```python
from build123d import *

# Parameters (mm, degrees)
F1_DEPTH = 30
F2_R     = 4.4
F3_R     = 4.4
F4_DEPTH = 25
F5_R     = 2
F6_R     = 2


# Not quite as in the source:
# - a feature names something its author has since deleted; it is built from what else it names


with BuildPart() as f1:
    # F0 (on Front) → F1 (new body)
    with BuildSketch(Plane.XZ):
        Polygon((90, -1), (90, 1), (70, 1), (70, 69), (-70, 69), (-70, 1), (-90, 1), (-90, -1), (-68, -1), (-68, 67), (68, 67), (68, -1), align=None)
    extrude(amount=F1_DEPTH)

    # F2 (on face) + F3 (on face) → F4 (cut)
    with BuildSketch(Plane.XY.offset(1)):
        with Locations((-80, -15)):
            Circle(F2_R)
        with Locations((80, -15)):
            Circle(F2_R)
    with BuildSketch(Plane.XY.offset(69)):
        with Locations((-25, -15)):
            Circle(F3_R)
        with Locations((25, -15)):
            Circle(F3_R)
    extrude(amount=-F4_DEPTH, mode=Mode.SUBTRACT)

    # F5
    f5_edges = [f1.edges().sort_by_distance(p)[0] for p in [
        (-70, -15, 69),
        (70, -15, 69),
    ]]
    fillet(f5_edges, radius=F5_R)

    # F6
    f6_edges = [f1.edges().sort_by_distance(p)[0] for p in [
        (68, -15, -1),
        (-68, -15, -1),
    ]]
    fillet(f6_edges, radius=F6_R)


solid = f1.part
```
Can you work these out from the model? Positions are in its coordinate system, mm. A direction names the side the tool comes from. Coordinates: 2 decimals unless noted, no trailing zeros. Order: outer loops, then holes, each group sorted by start corner. A loop starts at its lowest first (then second) coordinate and runs counter-clockwise, first axis right, second up.
1. I'm going to push flat-ended pins straight in: pin 1 (6 mm diameter, centred on x = -79, y = -13.5, fed in from +Z); pin 2 (8 mm diameter, centred on x = -80, y = -15, fed in from -Z); pin 3 (9 mm diameter, centred on y = -17, z = 29.5, fed in from +X); pin 4 (5 mm diameter, centred on x = -34.5, y = -6, fed in from -Z). Where does each tip first touch, or does it pass through?
2. Thinking about a two-plate mould opening in Y: for faces 4 (the face through (-22.635, -11.29, 68.014)), 5 (the face through (0, 0, 68)), 6 (the face through (-84.396, -14.807, 0.014)), 7 (the face through (-70, -15, 34)), which applies, +Y half, -Y half, draft (parallel to the pull), parting line (faces both ways), or undercut?
3. If we section it at B-B (y = -15): Give the number of separate pieces and of enclosed holes in the cut face, then the cut area to 3 significant figures.
4. For faces 1 (the face through (68, -15, 34)), 2 (the face through (85, -15, 1)), 3 (the face through (-75, -15, 1)), which set-ups out of +Z, -Z, +X, -X, +Y, -Y let a thin tool reach every point of the face, with its end or its side?
5. I need wall thicknesses on line 1 (X direction, y = -16, z = 18.5); line 2 (Y direction, x = 25, z = 68); line 3 (Z direction, x = -40, y = -24.25). Which ranges of each line are inside material? Lowest first, please.
6. If we section it at A-A (z = 60.5): Please give me the cut outline in (x, y), then the cut area to 3 significant figures.
7. If we section it at C-C (x = 80): Please give me the cut outline in (y, z), then the cut area to 3 significant figures.
8. If we section it at D-D (y = -5): Please give me the cut outline in (x, z).
Entries:
1. pin 1: stops at z = 1
1. pin 2: passes through
1. pin 3: stops at x = 70
1. pin 4: stops at z = 67
2. face 4: undercut
2. face 5: +Y half
2. face 6: undercut
2. face 7: draft
3. separate pieces: 5
3. enclosed holes: 0
3. area: 558 mm2
4. face 1: -Z, +Y, -Y
4. face 2: +Z, +X, +Y, -Y
4. face 3: +Z, -X, +Y, -Y
5. line 1: x = -70 to -68, 68 to 70
5. line 2: y = -30 to -19.4, -10.6 to 0
5. line 3: z = 67 to 69
6. outline: (-70, -30) - (-68, -30) - (-68, 0) - (-70, 0) - close; (68, -30) - (70, -30) - (70, 0) - (68, 0) - close
6. area: 120 mm2
7. outline: (-30, -1) - (-19.4, -1) - (-19.4, 1) - (-30, 1) - close; (-10.6, -1) - (0, -1) - (0, 1) - (-10.6, 1) - close
7. area: 42.4 mm2
8. outline: (-90, -1) - (-70, -1) arc R2 ccw to (-68, 1) - (-68, 67) - (68, 67) - (68, 1) arc R2 ccw to (70, -1) - (90, -1) - (90, 1) - (70, 1) - (70, 67) arc R2 ccw to (68, 69) - (-68, 69) arc R2 ccw to (-70, 67) - (-70, 1) - (-90, 1) - close
